```python
from build123d import *

# Parameters (mm, degrees)
SKETCH1_W           = 10.668
SKETCH1_H           = 7.112
BOSS_EXTRUDE1_DEPTH = 0.762
SKETCH2_W           = 1.8415
SKETCH2_H           = 5.842
BOSS_EXTRUDE2_DEPTH = 0.254
FILLET1_R           = 0.254


with BuildPart() as part:
    # Sketch1 → Boss-Extrude1 (new body)
    with BuildSketch(Plane.XY):
        with Locations((5.334, 3.556)):
            Rectangle(SKETCH1_W, SKETCH1_H)
    extrude(amount=BOSS_EXTRUDE1_DEPTH)

    # Sketch2 → Boss-Extrude2 (add)
    with BuildSketch(Plane.XY.offset(0.762)):
        with Locations((8.85825, 3.556)):
            Rectangle(SKETCH2_W, SKETCH2_H)
        with Locations((1.80975, 3.556)):
            Rectangle(SKETCH2_W, SKETCH2_H)
        with Locations((4.15925, 3.556)):
            Rectangle(SKETCH2_W, SKETCH2_H)
        with Locations((6.50875, 3.556)):
            Rectangle(SKETCH2_W, SKETCH2_H)
    extrude(amount=BOSS_EXTRUDE2_DEPTH)

    # Fillet1
    fillet1_edges = [part.edges().sort_by_distance(p)[0] for p in [
        (2.7305, 3.556, 1.016),
        (1.80975, 0.635, 1.016),
        (0.889, 3.556, 1.016),
        (1.80975, 6.477, 1.016),
        (5.08, 3.556, 1.016),
        (4.15925, 0.635, 1.016),
        (3.2385, 3.556, 1.016),
        (4.15925, 6.477, 1.016),
        (9.779, 3.556, 1.016),
        (8.85825, 0.635, 1.016),
        (7.9375, 3.556, 1.016),
        (8.85825, 6.477, 1.016),
        (7.4295, 3.556, 1.016),
        (6.50875, 0.635, 1.016),
        (5.588, 3.556, 1.016),
        (6.50875, 6.477, 1.016),
    ]]
    fillet(fillet1_edges, radius=FILLET1_R - 0.0001)  # a hair under: the kernel refuses the full size


solid = part.part
```
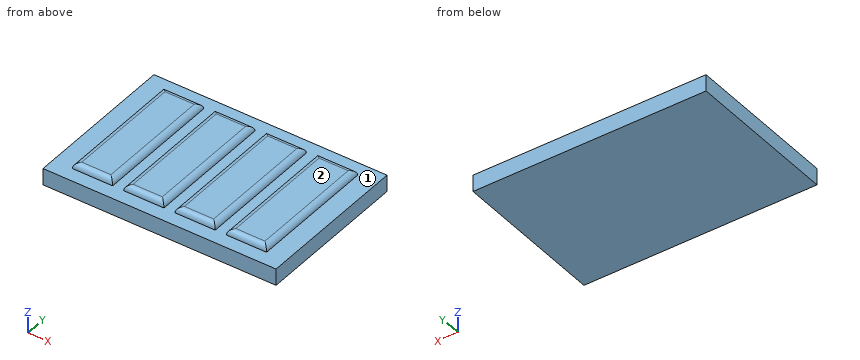
Source: CAD feature listing. Evaluate the final solid. Frame: model axes, mm. Face numbers are marked on the shaded views. Round coordinates to 2 decimals unless told otherwise and drop trailing zeros. Loops run counter-clockwise (first coordinate to the right, second up) from the corner with the lowest first, then second, coordinate; pieces in that order, holes last. Notation, with made-up numbers: M -17.75,9.5 L 39.25,9.5 A26 ccw 39.25,36.5 Z; hole C 69.25,-11 d4. An arc over 180 degrees is marked long. Put each result on its own line as item: value.
(1) Pull-direction query (X, two-part tool) for the marked faces 1 and 2; classes: released by +X, released by -X, zero draft, split by the parting line, or undercut.
Solutions:
face 1: undercut
face 2: zero draft
(2) Section C-C, the plane x = 0.75. Return loops of the section in (y, z).
Solutions:
outline: M 0,0 L 7.11,0 L 7.11,0.76 L 0,0.76 Z
(3) Ray query, line 1 (X direction, y = 3.25, z = 0.95); line 2 (Z direction, x = 9.5, y = 6.75); line 3 (Z direction, x = 5, y = 6.25). Return the intervals inside material, ascending. Write a range as [from, to].
Solutions:
line 1: [0.97, 2.65], [3.32, 5], [5.67, 7.35], [8.02, 9.7]
line 2: [0, 0.76]
line 3: [0, 0.95]
